Study the drawing (mm; zero at the part's minimum x, y, z) and answer. A direction names the side the tool comes from. Give positions to 0.01 mm unless a question says otherwise; leave off trailing zeros. Order: outer loops, then holes, each group sorted by start corner. A loop starts at its lowest first (then second) coordinate and runs counter-clockwise, first axis right, second up.
Item 1: A cutting plane is placed at D-D (x = 5.75). Write down the section's boundary in (y, z).
Item 2: The mould has two halves that part along Z. Classify the marked faces 3, 4 and 5: +Z half, -Z half, draft (parallel to the pull), parting line (faces both ways), or undercut.
Item 3: Find the intervals of material crossed by line 1 along X through (y, z) = (2.5, 6.35); line 2 along Z through (x, y) = (4.25, 12.7), in increasing order.
Item 4: Given pin 1 Ø4.5 at (y, z) = (12.7, 6.35) entering from -X, flat-ended and moving along its own axis, determine where the tip first touches the part or whether it passes through.
Item 5: Which of the six approach directions +Z, -Z, +X, -X, +Y, -Y give full straight-line access (tool end or side, diameter ignored) to the marked faces 1 and 2?
Item 6: A cutting plane is placed at A-A (y = 12.7). Write down the section's boundary in (x, z).
Item 7: A cutting plane is placed at B-B (z = 6.35). Write down the section's boundary in (x, y).
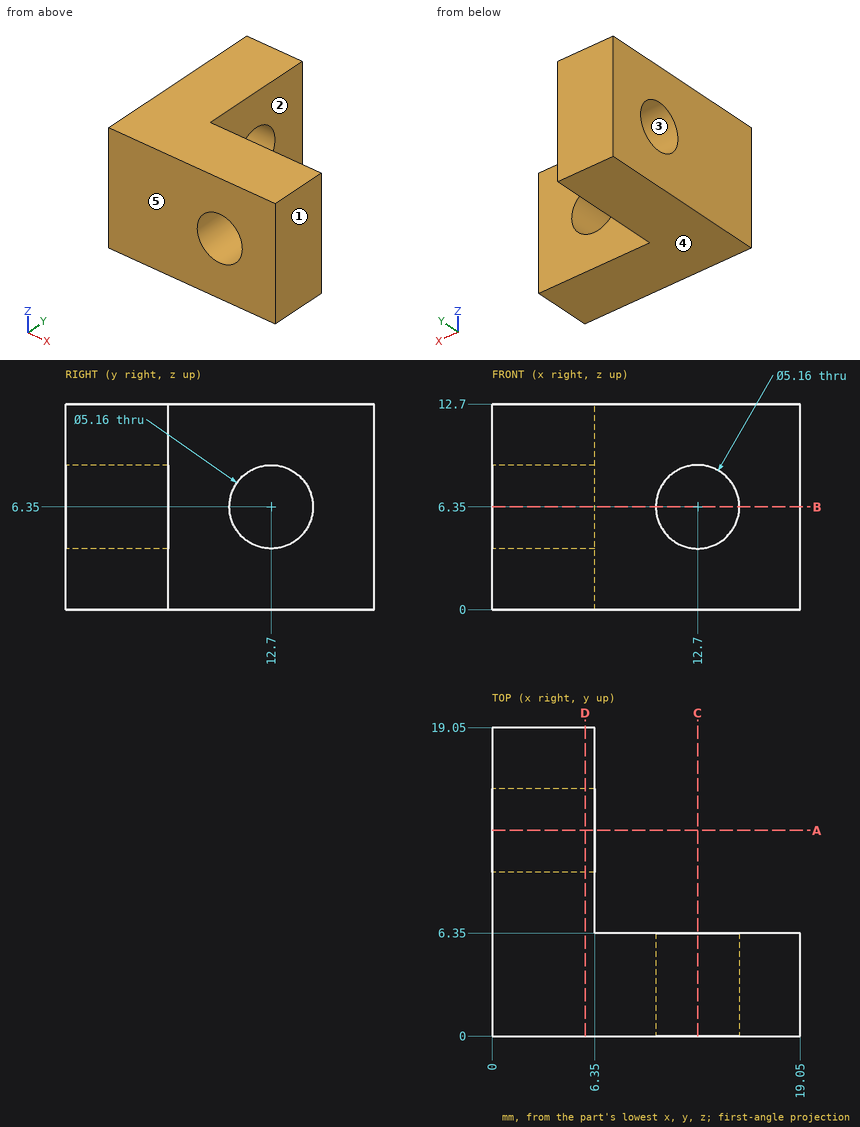
Response values:
1. outline: (0, 0) - (19.05, 0) - (19.05, 12.7) - (0, 12.7) - close; hole circle Ø5.16 at (12.7, 6.35)
2. face 3: undercut
2. face 4: -Z half
2. face 5: draft
3. line 1: x = 0 to 10.12, 15.28 to 19.05
3. line 2: z = 0 to 3.77, 8.93 to 12.7
4. pin 1: passes through
5. face 1: +Z, -Z, +X, +Y, -Y
5. face 2: +Z, -Z, +X, +Y
6. outline: (0, 0) - (6.35, 0) - (6.35, 3.77) - (0, 3.77) - close; (0, 8.93) - (6.35, 8.93) - (6.35, 12.7) - (0, 12.7) - close
7. outline: (0, 0) - (10.12, 0) - (10.12, 6.35) - (6.35, 6.35) - (6.35, 10.12) - (0, 10.12) - close; (0, 15.28) - (6.35, 15.28) - (6.35, 19.05) - (0, 19.05) - close; (15.28, 0) - (19.05, 0) - (19.05, 6.35) - (15.28, 6.35) - close
